Geometry check sheet. Reference: drawing and pictorial views, mm from the part's lowest x, y, z. A direction names the side the tool comes from. Round coordinates to 2 decimals unless told otherwise and drop trailing zeros. Write each loop counter-clockwise with the first axis right and the second up, starting at its lowest first coordinate (ties: lowest second). Pieces come first, ordered by that corner, then holes. Notation, with made-up numbers: (-14, -24.75) -> (-3, -24.75) arc R17 cw to (-3, -19.75) -> close; hole circle Ø10 at (26.25, 7). An arc over 180 degrees is marked (long way). Answer as a JSON object with one key per item and string values. Group by question number.
(1) Sectioned sample at C-C on y = 9.8. Record the cut outline in (x, z), and give its area (3 significant figures).
(2) Gauge pin test, flat ends, axial feed: pin 1 Ø3.5 at (x, y) = (4, 9) entering from +Z; pin 2 Ø1 at (x, y) = (7.5, 7.5) entering from -Z; pin 3 Ø4 at (y, z) = (2.5, 8) entering from +X. Record the tip position at first contact, or that the pin passes through.
(3) Draft check along X on the marked faces 1, 2 and 3. Enter one of: released by +X, released by -X, zero draft, split by the parting line, or undercut.
(4) Scan lines: L1, parallel to X at y = 4.75, z = 6; L2, parallel to Z at x = 1.25, y = 11.5; L3, parallel to Z at x = 7, y = 6.5. Record each from-to range of solid material in increasing order. Write a range as from..to.
(5) Set-up check for the marked faces 4, 5, 6 and 7: record each of +Z, -Z, +X, -X, +Y, -Y from which the full face is reachable in a straight line by a thin tool's end or side.
(6) Sectioned sample at D-D on x = 2.3. Record the cut outline in (y, z), and give its area (3 significant figures).
(7) Sectioned sample at A-A on x = 8. Record the cut outline in (y, z).
(8) Sectioned sample at B-B on z = 9.75. Record the cut outline in (x, y), and give its area (3 significant figures).
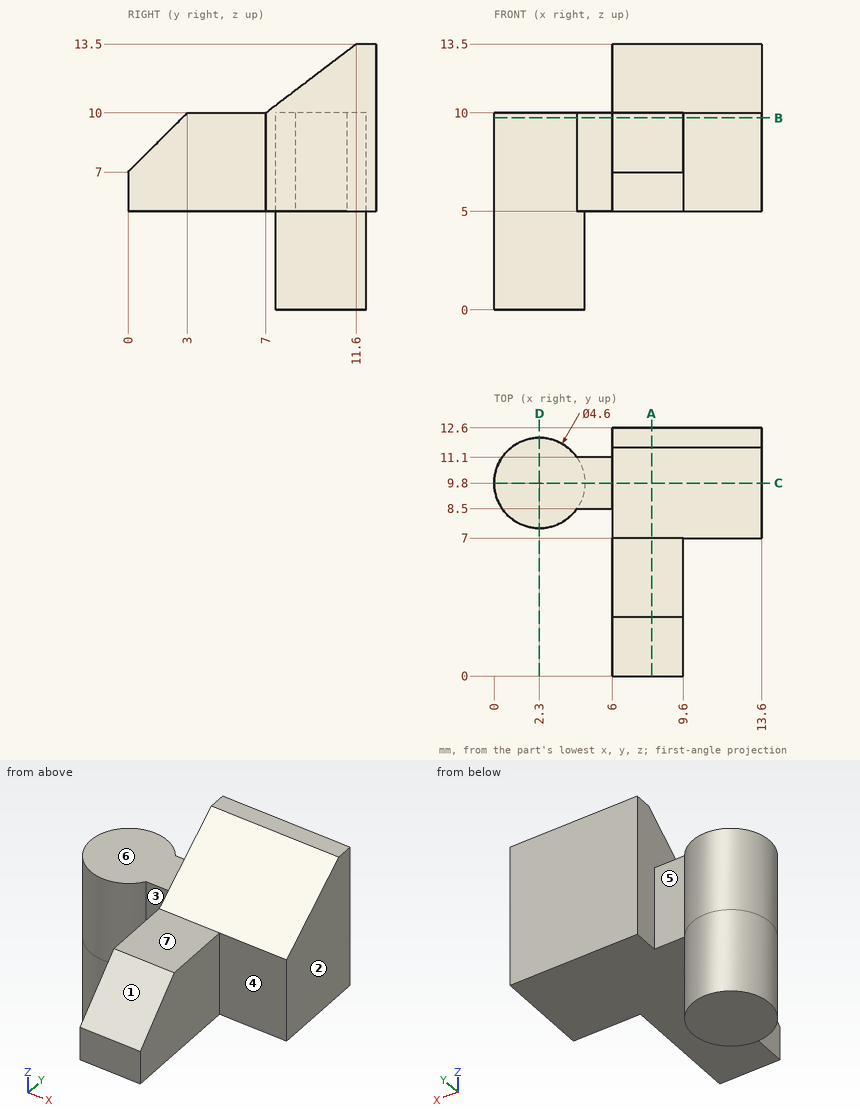
Computed values:
{
 "1": {"outline": "(0, 0) -> (4.6, 0) -> (4.6, 5) -> (13.6, 5) -> (13.6, 12.13) -> (6, 12.13) -> (6, 10) -> (0, 10) -> close", "area": "107 mm2"},
 "2": {"pin 1": "z = 10", "pin 2": "z = 5", "pin 3": "x = 9.6"},
 "3": {"face 1": "zero draft", "face 2": "released by +X", "face 3": "undercut"},
 "4": {"L1": "6..9.6", "L2": "0..10", "L3": "5..10"},
 "5": {"face 4": "+Z, -Z, +X, -Y", "face 5": "+Z, -Z, +Y", "face 6": "+Z, -X, +Y, -Y", "face 7": "+Z, +X, -X, -Y"},
 "6": {"outline": "(7.5, 0) -> (12.1, 0) -> (12.1, 10) -> (7.5, 10) -> close", "area": "46.0 mm2"},
 "7": {"outline": "(0, 5) -> (12.6, 5) -> (12.6, 13.5) -> (11.6, 13.5) -> (7, 10) -> (3, 10) -> (0, 7) -> close"},
 "8": {"outline": "(4.2, 8.5) -> (6, 8.5) -> (6, 2.75) -> (9.6, 2.75) -> (9.6, 7) -> (13.6, 7) -> (13.6, 12.6) -> (6, 12.6) -> (6, 11.1) -> (4.2, 11.1) arc R2.3 ccw (long way) to start", "area": "78.5 mm2"}
}
